from build123d import *

# Parameters (mm, degrees)
F0_R          = 1.65
F1_DEPTH      = 10
F0_R_2        = 2.6
F2_DEPTH      = 4
F0_R_3        = 2
F3_DEPTH      = 4.5
F5_R          = 3
F6_DEPTH      = 2
F6_TAPER      = 45
F6_DEPTH_BACK = 2
F6_TAPER_BACK = -45
F7_DEPTH      = 25
F5_W          = 2
F5_H          = 1.75
F8_DEPTH      = 25


with BuildPart() as f1:
    # F0 (on Top) → F1 (new body)
    with BuildSketch(Plane.XY):
        with BuildLine():
            ThreePointArc((14.7096774194, -18.9096026482), (12.824730257, -13.2432475097), (18.7276803364, -14.1464566331))
            Line((18.7276803364, -14.1464566331), (13.8684226679, -2.5589960389))
            ThreePointArc((13.8684226679, -2.5589960389), (10.9739243006, -5.1335779779), (7.1001902802, -5.1614652017))
            ThreePointArc((7.1001902802, -5.1614652017), (4.6080160796, -11.0514527236), (-1.6067478385, -12.5612853954))
            Line((-1.6067478385, -12.5612853954), (-14.1451612903, -9.6549668888))
            ThreePointArc((-14.1451612903, -9.6549668888), (-17.6142039843, -9.8848293425), (-20.3733971724, -12))
            Line((-20.3733971724, -12), (-18.3428150172, -13.4583333333))
            ThreePointArc((-18.3428150172, -13.4583333333), (-16.7332856575, -12.2244837831), (-14.7096774194, -12.0903973518))
            Line((-14.7096774194, -12.0903973518), (14.7096774194, -18.9096026482))
        make_face()
        with BuildLine():
            ThreePointArc((14.7096774194, -18.9096026482), (17.6775985589, -18.2400847644), (19, -15.5))
            ThreePointArc((19, -15.5), (18.9312447579, -14.8096671735), (18.7276803364, -14.1464566331))
            ThreePointArc((18.7276803364, -14.1464566331), (12.824730257, -13.2432475097), (14.7096774194, -18.9096026482))
        make_face()
        with Locations((15.5, -15.5)):
            Circle(F0_R, mode=Mode.SUBTRACT)
    extrude(amount=F1_DEPTH)

    # F0 (on Top) → F2 (join)
    with BuildSketch(Plane.XY):
        with BuildLine():
            ThreePointArc((7.1001902802, -5.1614652017), (10.9739243006, -5.1335779779), (13.8684226679, -2.5589960389))
            Line((13.8684226679, -2.5589960389), (12.2276803364, 1.3535433669))
            ThreePointArc((12.2276803364, 1.3535433669), (7.3899296254, 3.1076797436), (6.0326682233, -1.856055529))
            ThreePointArc((6.0326682233, -1.856055529), (6.7712204508, -3.4426205691), (7.1001902802, -5.1614652017))
        make_face()
        with Locations((9, 0)):
            Circle(F0_R_2, mode=Mode.SUBTRACT)
    extrude(amount=F2_DEPTH)

    # F0 (on Top) → F3 (join)
    with BuildSketch(Plane.XY):
        with Locations((9, 0)):
            Circle(F0_R_2)
        with Locations((9, 0)):
            Circle(F0_R_3, mode=Mode.SUBTRACT)
    extrude(amount=F3_DEPTH)

    # F5 (on offset) → F6 (join, two sides)
    with BuildSketch(Plane.XZ.offset(9.5)) as f6_sk:
        with Locations((-15.5, 5)):
            Circle(F5_R)
    extrude(amount=-F6_DEPTH, taper=F6_TAPER)
    extrude(f6_sk.sketch, amount=F6_DEPTH_BACK, taper=F6_TAPER_BACK)

    # F5 (on offset) → F7 (cut)
    with BuildSketch(Plane.XZ.offset(9.5)):
        with BuildLine():
            ThreePointArc((4.5000000108, 6.25), (3.6161165273, 5.8838834803), (3.25, 5))
            ThreePointArc((3.25, 5), (4.5, 3.75), (5.75, 5))
            ThreePointArc((5.75, 5), (5.3838834803, 5.8838834727), (4.5000000108, 6.25))
        make_face()
        with BuildLine():
            ThreePointArc((3.25, 7.5), (3.6161165273, 6.6161165197), (4.5000000108, 6.25))
            ThreePointArc((4.5000000108, 6.25), (5.3838834803, 6.6161165273), (5.75, 7.5))
            ThreePointArc((5.75, 7.5), (4.5, 8.75), (3.25, 7.5))
        make_face()
        with BuildLine():
            Line((3.25, 7.5), (3.25, 5))
            ThreePointArc((3.25, 5), (3.6161165273, 5.8838834803), (4.5000000108, 6.25))
            ThreePointArc((4.5000000108, 6.25), (3.6161165273, 6.6161165197), (3.25, 7.5))
        make_face()
        with BuildLine():
            ThreePointArc((4.5000000108, 6.25), (5.3838834803, 5.8838834727), (5.75, 5))
            Line((5.75, 5), (5.75, 7.5))
            ThreePointArc((5.75, 7.5), (5.3838834803, 6.6161165273), (4.5000000108, 6.25))
        make_face()
    extrude(amount=F7_DEPTH, mode=Mode.SUBTRACT)

    # F5 (on offset) → F8 (cut)
    with BuildSketch(Plane.XZ.offset(9.5)):
        with Locations((5.5, 0.875)):
            Rectangle(F5_W, F5_H)
    extrude(amount=-F8_DEPTH, mode=Mode.SUBTRACT)


solid = f1.part
The listing builds one solid part. Answer for the finished solid, in the listing's coordinates (mm). A direction names the side the tool comes from. Coordinates: 2 decimals unless noted, no trailing zeros. Loops run counter-clockwise (first coordinate to the right, second up) from the corner with the lowest first, then second, coordinate; pieces in that order, holes last. Notation, with made-up numbers: (71.5, 82) -> (111.5, 82) arc R32 ccw to (111.5, 108) -> close; hole circle Ø11 at (87, 49.25). An arc over 180 degrees is marked (long way). Write item = value, one per line. Start each with the question number.
1) A cutting plane is placed at D-D (x = 4.5). Give the vertices of the cut face in (y, z), then the cut area to 3 significant figures.
2) A tool of negligible diameter and unlimited length cuts with its end or side. For faces 1 (the face through (10, -3, 4)), 2 (the face through (-16, -7.5, 5)), 3 (the face through (4.953, -14.057, 8.665)), from which of +Z, -Z, +X, -X, +Y, -Y can it reach the whole face along a straight path? Write none if from no direction.
3) Straight lines are drawn through the part: line 1 (Y direction, x = 0, z = 2); line 2 (Y direction, x = 15.5, z = 7); line 3 (Y direction, x = 9, z = 2). For each, find the intervals that lie inside material, in ascending order. Write a range as from..to.
4) A cutting plane is placed at A-A (z = 0.75). Give the vertices of the cut face in (x, y).
5) Given pin 1 Ø4 at (x, y) = (9.5, -1) entering from +Z; pin 2 Ø0.9 at (y, z) = (-1.5, 1.5) entering from -X; pin 3 Ø0.5 at (y, z) = (-9, 1) entering from -X; pin 4 Ø6.5 at (x, y) = (9.5, -3) entering from +Z, each flat-ended and moving along its own axis, determine where each tip first touches the part or whether it passes through.
6) A cutting plane is placed at C-C (y = 0). Give the vertices of the cut face in (x, z), then the cut area to 3 significant figures.
7) A cutting plane is placed at B-B (x = 15.5). Give the vertices of the cut face in (y, z), then the cut area to 3 significant figures.
8) The mould has two halves that part along X. Classify faces 4 (the face through (-20.1, -11.65, 4.93)), 5 (the face through (4.902, -14.057, 3.816)), 6 (the face through (8.693, 3.487, 2.416)), 7 (the face through (6.5, -9, 1)): released by +X, released by -X, zero draft, split by the parting line, or undercut.
Responses:
q1.outline = (-16.54, 0) -> (-11.14, 0) -> (-11.14, 3.75) -> (-16.54, 3.75) -> close; (-16.54, 8.75) -> (-11.14, 8.75) -> (-11.14, 10) -> (-16.54, 10) -> close
q1.area = 27.0 mm²
q2.face_1 = +Z
q2.face_2 = +Z, -Z, -X, +Y
q2.face_3 = +Y, -Y
q3.line_1 = -15.5..-12.75
q3.line_2 = -19..-17.15, -13.85..-6.45
q3.line_3 = -17.59..-2, 2..3.5
q4.outline = (-20.37, -12) -> (-18.34, -13.46) arc R3.5 cw to (-14.71, -12.09) -> (14.71, -18.91) arc R3.5 ccw to (18.73, -14.15) -> (12.23, 1.35) arc R3.5 ccw to (6.5, 2.45) -> (6.5, -2.73) arc R7.12 cw to (6.5, -8.52) -> (6.5, -9.5) -> (5.97, -9.5) arc R7.12 cw to (-1.61, -12.56) -> (-14.15, -9.65) arc R6 ccw to start; hole circle Ø4 at (9, 0); hole circle Ø3.3 at (15.5, -15.5)
q5.pin_1 = 4.5
q5.pin_2 = 5.69
q5.pin_3 = 6.5
q5.pin_4 = 10
q6.outline = (5.5, 1.75) -> (6.5, 1.75) -> (6.5, 0) -> (7, 0) -> (7, 4.5) -> (6.4, 4.5) -> (6.4, 4) -> (5.5, 4) -> close; (11, 0) -> (12.8, 0) -> (12.8, 4) -> (11.6, 4) -> (11.6, 4.5) -> (11, 4.5) -> close
q6.area = 12.0 mm²
q7.outline = (-19, 0) -> (-17.15, 0) -> (-17.15, 10) -> (-19, 10) -> close; (-13.85, 0) -> (-6.45, 0) -> (-6.45, 10) -> (-13.85, 10) -> close
q7.area = 92.5 mm²
q8.face_4 = undercut
q8.face_5 = undercut
q8.face_6 = split by the parting line
q8.face_7 = released by -X
